from build123d import *

# Parameters (mm, degrees)
F0_R     = 12.7
F0_R_2   = 6.35
F1_DEPTH = 6.35
F2_W     = 384.192481637
F2_H     = 305.0564825535
F3_DEPTH = 342.9


with BuildPart() as f1:
    # F0 (on Top) → F1 (new body)
    with BuildSketch(Plane.XY):
        Polygon((0, 20.4046759754), (0, 99.420234561), (-200.6414681673, 99.420234561), (-200.6414681673, -93.7068536878), (-200.6414681673, -249.9808818102), (0, -249.9808818102), (0, -172.3671704531), (-84.5718756318, -172.3671704531), (-84.5718756318, 20.4046759754), align=None)
        with Locations((-149.8414681673, -186.0281676054)):
            Circle(F0_R, mode=Mode.SUBTRACT)
        with Locations((-149.8410850763, 35.5835556984)):
            Circle(F0_R, mode=Mode.SUBTRACT)
        with BuildLine():
            ThreePointArc((528.9263289283, -457.4688246387), (513.3995365217, -448.3073763574), (498.0855940313, -438.7944071863))
            ThreePointArc((498.0855940313, -438.7944071863), (450.3295426137, -436.1242750207), (408.4167574662, -459.1696323397))
            ThreePointArc((408.4167574662, -459.1696323397), (386.971113082, -494.1413749169), (383.9916826006, -535.0566707847))
            ThreePointArc((383.9916826006, -535.0566707847), (476.7448379257, -607.1755616667), (556.3054700156, -520.7210183144))
            ThreePointArc((556.3054700156, -520.7210183144), (549.1669902089, -486.2592374134), (528.9263289283, -457.4688246387))
        make_face()
        with Locations((413.9536619186, -520.7210183144)):
            Circle(F0_R_2, mode=Mode.SUBTRACT)
        with Locations((469.5522487164, -574.6076107025)):
            Circle(F0_R_2, mode=Mode.SUBTRACT)
        with BuildLine():
            ThreePointArc((493.1213777738, -520.7210183144), (460.4958391633, -542.4807354663), (452.9429486617, -503.9987279144))
            ThreePointArc((452.9429486617, -503.9987279144), (478.6086582694, -498.9613011624), (493.1213777738, -520.7210183144))
        make_face(mode=Mode.SUBTRACT)
        with Locations((527.7953147888, -520.7210183144)):
            Circle(F0_R_2, mode=Mode.SUBTRACT)
        with Locations((469.5522487164, -457.730203867)):
            Circle(F0_R_2, mode=Mode.SUBTRACT)
        with BuildLine():
            ThreePointArc((498.0855940313, -438.7944071863), (323.9779289887, -288.1314492402), (200.6414681673, -93.7068536878))
            Line((200.6414681673, -93.7068536878), (200.6414681673, -249.9808818102))
            Line((200.6414681673, -249.9808818102), (408.4167574662, -459.1696323397))
            ThreePointArc((408.4167574662, -459.1696323397), (450.3295426137, -436.1242750207), (498.0855940313, -438.7944071863))
        make_face()
        Polygon((200.6414681673, 99.420234561), (0, 99.420234561), (0, 20.4046759754), (84.5718756318, 20.4046759754), (84.5718756318, -172.3671704531), (0, -172.3671704531), (0, -249.9808818102), (200.6414681673, -249.9808818102), (200.6414681673, -93.7068536878), align=None)
        with Locations((149.8414681673, -186.0281676054)):
            Circle(F0_R, mode=Mode.SUBTRACT)
        with Locations((149.8410850763, 35.5835556984)):
            Circle(F0_R, mode=Mode.SUBTRACT)
        with BuildLine():
            Line((355.8921389085, 267.9402017142), (200.6414681673, 99.420234561))
            Line((200.6414681673, 99.420234561), (200.6414681673, -93.7068536878))
            ThreePointArc((200.6414681673, -93.7068536878), (279.3415917253, 99.1204583435), (427.1100518471, 245.8874979214))
            ThreePointArc((427.1100518471, 245.8874979214), (389.0113531334, 248.873373327), (355.8921389085, 267.9402017142))
        make_face()
        with BuildLine():
            ThreePointArc((330.8906401246, 354.2550166966), (195.3973793112, 187.9463252543), (0, 99.420234561))
            Line((0, 99.420234561), (200.6414681673, 99.420234561))
            Line((200.6414681673, 99.420234561), (355.8921389085, 267.9402017142))
            ThreePointArc((355.8921389085, 267.9402017142), (331.3444814273, 307.6081646876), (330.8906401246, 354.2550166966))
        make_face()
        with BuildLine():
            Line((-200.6414681673, 99.420234561), (0, 99.420234561))
            ThreePointArc((0, 99.420234561), (-195.3973793112, 187.9463252543), (-330.8906401246, 354.2550166966))
            ThreePointArc((-330.8906401246, 354.2550166966), (-328.6653224016, 343.0974003758), (-327.9192726354, 331.7445218563))
            ThreePointArc((-327.9192726354, 331.7445218563), (-335.2196571274, 296.9110877867), (-355.8921389085, 267.9402017142))
            Line((-355.8921389085, 267.9402017142), (-200.6414681673, 99.420234561))
        make_face()
        with BuildLine():
            Line((-200.6414681673, -93.7068536878), (-200.6414681673, 99.420234561))
            Line((-200.6414681673, 99.420234561), (-355.8921389085, 267.9402017142))
            ThreePointArc((-355.8921389085, 267.9402017142), (-389.0113531334, 248.873373327), (-427.1100518471, 245.8874979214))
            ThreePointArc((-427.1100518471, 245.8874979214), (-279.3415917253, 99.1204583435), (-200.6414681673, -93.7068536878))
        make_face()
        with BuildLine():
            Line((-200.6414681673, -249.9808818102), (-200.6414681673, -93.7068536878))
            ThreePointArc((-200.6414681673, -93.7068536878), (-323.9779289887, -288.1314492402), (-498.0855940313, -438.7944071863))
            ThreePointArc((-498.0855940313, -438.7944071863), (-450.3295426137, -436.1242750207), (-408.4167574662, -459.1696323397))
            Line((-408.4167574662, -459.1696323397), (-200.6414681673, -249.9808818102))
        make_face()
        with BuildLine():
            ThreePointArc((-408.4167574662, -459.1696323397), (-450.3295426137, -436.1242750207), (-498.0855940313, -438.7944071863))
            ThreePointArc((-498.0855940313, -438.7944071863), (-513.3995365217, -448.3073763574), (-528.9263289283, -457.4688246387))
            ThreePointArc((-528.9263289283, -457.4688246387), (-510.4961307794, -597.2044801045), (-383.9916826006, -535.0566707847))
            ThreePointArc((-383.9916826006, -535.0566707847), (-383.097705364, -527.9136075237), (-382.7990274171, -520.7210183144))
            ThreePointArc((-382.7990274171, -520.7210183144), (-389.4591085374, -487.3861971499), (-408.4167574662, -459.1696323397))
        make_face()
        with Locations((-469.5522487164, -574.6076107025)):
            Circle(F0_R_2, mode=Mode.SUBTRACT)
        with Locations((-527.7953147888, -520.7210183144)):
            Circle(F0_R_2, mode=Mode.SUBTRACT)
        with BuildLine():
            ThreePointArc((-445.9831196589, -520.7210183144), (-491.3119658683, -529.7774278674), (-452.9429486617, -503.9987279144))
            ThreePointArc((-452.9429486617, -503.9987279144), (-447.7925315644, -511.6646087613), (-445.9831196589, -520.7210183144))
        make_face(mode=Mode.SUBTRACT)
        with Locations((-413.9536619186, -520.7210183144)):
            Circle(F0_R_2, mode=Mode.SUBTRACT)
        with Locations((-469.5522487164, -457.730203867)):
            Circle(F0_R_2, mode=Mode.SUBTRACT)
        with BuildLine():
            ThreePointArc((342.2890075184, 379.5645208111), (336.7772209347, 366.8253727446), (330.8906401246, 354.2550166966))
            ThreePointArc((330.8906401246, 354.2550166966), (331.3444814273, 307.6081646876), (355.8921389085, 267.9402017142))
            ThreePointArc((355.8921389085, 267.9402017142), (389.0113531334, 248.873373327), (427.1100518471, 245.8874979214))
            ThreePointArc((427.1100518471, 245.8874979214), (480.2663946412, 274.9681042527), (501.4257152339, 331.7445218563))
            ThreePointArc((501.4257152339, 331.7445218563), (439.6386789688, 414.8276790582), (342.2890075184, 379.5645208111))
        make_face()
        with Locations((414.6724939346, 284.5172584057)):
            Circle(F0_R_2, mode=Mode.SUBTRACT)
        with Locations((360.8275949955, 331.7445218563)):
            Circle(F0_R_2, mode=Mode.SUBTRACT)
        with BuildLine():
            ThreePointArc((438.2416229921, 331.7445218563), (424.1360468818, 310.1587624269), (398.7030376666, 314.4101539409))
            ThreePointArc((398.7030376666, 314.4101539409), (405.2089409875, 353.3302812857), (438.2416229921, 331.7445218563))
        make_face(mode=Mode.SUBTRACT)
        with Locations((414.6724939346, 387.7336978912)):
            Circle(F0_R_2, mode=Mode.SUBTRACT)
        with Locations((464.0439748764, 331.7445218563)):
            Circle(F0_R_2, mode=Mode.SUBTRACT)
        with BuildLine():
            ThreePointArc((-327.9192726354, 331.7445218563), (-328.6653224016, 343.0974003758), (-330.8906401246, 354.2550166966))
            ThreePointArc((-330.8906401246, 354.2550166966), (-336.7772209347, 366.8253727445), (-342.2890075184, 379.5645208111))
            ThreePointArc((-342.2890075184, 379.5645208111), (-487.9238775271, 378.2241540363), (-427.1100518471, 245.8874979214))
            ThreePointArc((-427.1100518471, 245.8874979214), (-389.0113531334, 248.873373327), (-355.8921389085, 267.9402017142))
            ThreePointArc((-355.8921389085, 267.9402017142), (-335.2196571274, 296.9110877867), (-327.9192726354, 331.7445218563))
        make_face()
        with Locations((-414.6724939346, 284.5172584057)):
            Circle(F0_R_2, mode=Mode.SUBTRACT)
        with Locations((-464.0439748764, 331.7445218563)):
            Circle(F0_R_2, mode=Mode.SUBTRACT)
        with BuildLine():
            ThreePointArc((-391.1033648772, 331.7445218563), (-393.0867345053, 322.2809689092), (-398.7030376666, 314.4101539409))
            ThreePointArc((-398.7030376666, 314.4101539409), (-436.258253364, 341.2080748035), (-391.1033648772, 331.7445218563))
        make_face(mode=Mode.SUBTRACT)
        with Locations((-360.8275949955, 331.7445218563)):
            Circle(F0_R_2, mode=Mode.SUBTRACT)
        with Locations((-414.6724939346, 387.7336978912)):
            Circle(F0_R_2, mode=Mode.SUBTRACT)
        with BuildLine():
            ThreePointArc((-383.9916826006, -535.0566707847), (-215.6935374643, -360.5984288821), (0, -249.9808818102))
            Line((0, -249.9808818102), (-200.6414681673, -249.9808818102))
            Line((-200.6414681673, -249.9808818102), (-408.4167574662, -459.1696323397))
            ThreePointArc((-408.4167574662, -459.1696323397), (-389.4591085374, -487.3861971499), (-382.7990274171, -520.7210183144))
            ThreePointArc((-382.7990274171, -520.7210183144), (-383.097705364, -527.9136075237), (-383.9916826006, -535.0566707847))
        make_face()
        with BuildLine():
            Line((408.4167574662, -459.1696323397), (200.6414681673, -249.9808818102))
            Line((200.6414681673, -249.9808818102), (0, -249.9808818102))
            ThreePointArc((0, -249.9808818102), (215.6935374643, -360.5984288821), (383.9916826006, -535.0566707847))
            ThreePointArc((383.9916826006, -535.0566707847), (386.971113082, -494.1413749169), (408.4167574662, -459.1696323397))
        make_face()
    extrude(amount=F1_DEPTH)

    # F2 (on Top) → F3 (join)
    with BuildSketch(Plane.XY):
        with Locations((-1.2763813138, -83.0007791519)):
            Rectangle(F2_W, F2_H)
    extrude(amount=F3_DEPTH)


solid = f1.part
Can you work these out from the model? Positions are in its coordinate system, mm. A direction names the side the tool comes from. Coordinates: 2 decimals unless noted, no trailing zeros. Loops run counter-clockwise (first coordinate to the right, second up) from the corner with the lowest first, then second, coordinate; pieces in that order, holes last. Notation, with made-up numbers: M 53,48 L 103,48 A21 ccw 103,73 Z; hole C 12.5,43 d7. An arc over 180 degrees is marked long. Return JSON: item names as keys, results as strings. Group by question number.
Item 1: Thinking about a two-plate mould opening in Y: for faces 4 (the cylindrical face through (489.192, 376.163, 3.131)), 5 (the flat face through (-4, 69.527, 172)), 6 (the flat face through (190.82, -85, 172)), which applies, released by +Y, released by -Y, zero draft, split by the parting line, or undercut?
Item 2: On a 3-axis mill with a long thin cutter (end or side, diameter ignored), from which of +Z, -Z, +X, -X, +Y, -Y can I reach the whole of each face in a straight line? I mean faces 1 (the cylindrical face through (277.72, 96.674, 3.131)), 2 (the cylindrical face through (212.95, -358.57, 3.13)), 3 (the flat face through (-193.373, -85, 172)). Say none if no direction works.
Item 3: Imagine slicing it at D-D (z = 135). Please give me the cut outline in (x, y).
Item 4: Imagine slicing it at A-A (x = 235). Please give me the cut outline in (y, z), and give its area (3 significant figures).
Item 5: Imagine slicing it at C-C (x = 14.5). Please give me the cut outline in (y, z).
Item 6: Imagine slicing it at B-B (y = -400). Please give me the cut outline in (x, z), and give its area (3 significant figures).
Item 7: If I drill on L1, parallel to X at y = -144.5, z = 33.5; L2, parallel to Z at x = -490, y = -507.5; L3, parallel to Y at x = -105.5, z = 119.5, over which ranges is the centre line in solid material (lowest first)? Write a range as from..to.
Item 8: I'm going to push flat-ended pins straight in: pin 1 Ø16.5 at (x, y) = (-464.04, 331.74) entering from +Z; pin 2 Ø16.5 at (x, y) = (-414.67, 284.52) entering from -Z; pin 3 Ø12 at (x, z) = (-117, 71) entering from -Y; pin 4 Ø7.5 at (x, y) = (-413.95, -520.72) entering from -Z. Where does each tip first touch, or does it pass through?
Verdict:
{
 "1": {"face 4": "undercut", "face 5": "released by +Y", "face 6": "zero draft"},
 "2": {"face 1": "+Z, -Z, +X", "face 2": "+Z, -Z, -Y", "face 3": "+Z, -X, +Y, -Y"},
 "3": {"outline": "M -193.37,-235.53 L 190.82,-235.53 L 190.82,69.53 L -193.37,69.53 Z"},
 "4": {"outline": "M -375.43,0 L -161.78,0 L -161.78,6.35 L -375.43,6.35 Z; M 17.84,0 L 222.13,0 L 222.13,6.35 L 17.84,6.35 Z", "area": "2,650 mm^2"},
 "5": {"outline": "M -254.78,0 L 102.52,0 L 102.52,6.35 L 69.53,6.35 L 69.53,342.9 L -235.53,342.9 L -235.53,6.35 L -254.78,6.35 Z"},
 "6": {"outline": "M -442.59,0 L -264.32,0 L -264.32,6.35 L -442.59,6.35 Z; M 264.32,0 L 442.59,0 L 442.59,6.35 L 264.32,6.35 Z", "area": "2,260 mm^2"},
 "7": {"L1": "x = -193.37..190.82", "L2": "z = 0..6.35", "L3": "y = -235.53..69.53"},
 "8": {"pin 1": "stops at z = 6.35", "pin 2": "stops at z = 0", "pin 3": "stops at y = -235.53", "pin 4": "passes through"}
}
